Drawing for the job (mm, zero at the part's lowest x, y, z). A direction names the side the tool comes from. Round coordinates to 2 decimals unless told otherwise and drop trailing zeros. Write each loop counter-clockwise with the first axis right and the second up, starting at its lowest first coordinate (ties: lowest second). Pieces come first, ordered by that corner, then holes.
Item 1: Band-saw the part on B-B, the plane y = 2.5. Write the cut outline in (x, z) (1 decimal).
Item 2: Band-saw the part on C-C, the plane x = 14.75. Write the cut outline in (y, z).
Item 3: Band-saw the part on A-A, the plane x = 8. Write the cut outline in (y, z).
Item 4: Band-saw the part on D-D, the plane y = 1. Write the cut outline in (x, z).
Item 5: Drop a flat-ended pin along its axis: pin 1 Ø1 at (x, y) = (3.94, 5.79) entering from -Z. Give the stop position or say it passes through.
Item 6: Wall check: probe 1 along Z at (x, y) = (12.75, 10.75); probe 2 along Y at (x, z) = (3.25, 1.5) (1 decimal); probe 3 along X at (y, z) = (2.75, 12.25). Give the ranges that are in metal, low to high.
Item 7: 3-axis set-ups, long thin cutter, end or side, ignore diameter. For the marked faces 1 and 2: which of +Z, -Z, +X, -X, +Y, -Y reach the whole face in a straight line?
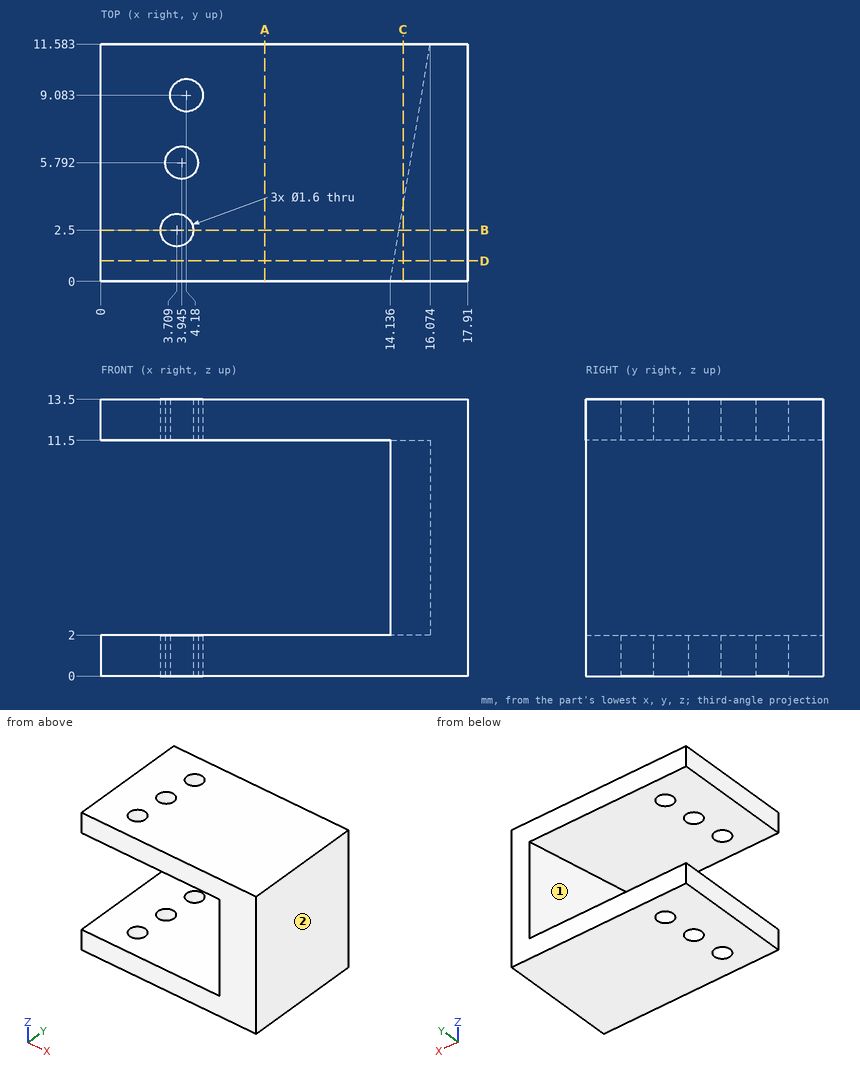
Results:
1. outline: (0, 0) - (2.9, 0) - (2.9, 2) - (0, 2) - close; (0, 11.5) - (2.9, 11.5) - (2.9, 13.5) - (0, 13.5) - close; (4.5, 0) - (17.9, 0) - (17.9, 13.5) - (4.5, 13.5) - (4.5, 11.5) - (14.6, 11.5) - (14.6, 2) - (4.5, 2) - close
2. outline: (0, 0) - (11.58, 0) - (11.58, 2) - (3.67, 2) - (3.67, 11.5) - (11.58, 11.5) - (11.58, 13.5) - (0, 13.5) - close
3. outline: (0, 0) - (11.58, 0) - (11.58, 2) - (0, 2) - close; (0, 11.5) - (11.58, 11.5) - (11.58, 13.5) - (0, 13.5) - close
4. outline: (0, 0) - (17.91, 0) - (17.91, 13.5) - (0, 13.5) - (0, 11.5) - (14.3, 11.5) - (14.3, 2) - (0, 2) - close
5. pin 1: passes through
6. probe 1: z = 0 to 2, 11.5 to 13.5
6. probe 2: y = 0 to 1.8, 3.2 to 5.4, 6.2 to 11.6
6. probe 3: x = 0 to 2.95, 4.47 to 17.91
7. face 1: -X, +Y
7. face 2: +Z, -Z, +X, +Y, -Y
